Input: dimensioned drawing with shaded views. Units: mm. Origin: part minimum x, y, z. A direction names the side the tool comes from. Coordinates: 2 decimals unless noted, no trailing zeros. Order: outer loops, then holes, each group sorted by start corner. A loop starts at its lowest first (then second) coordinate and runs counter-clockwise, first axis right, second up.
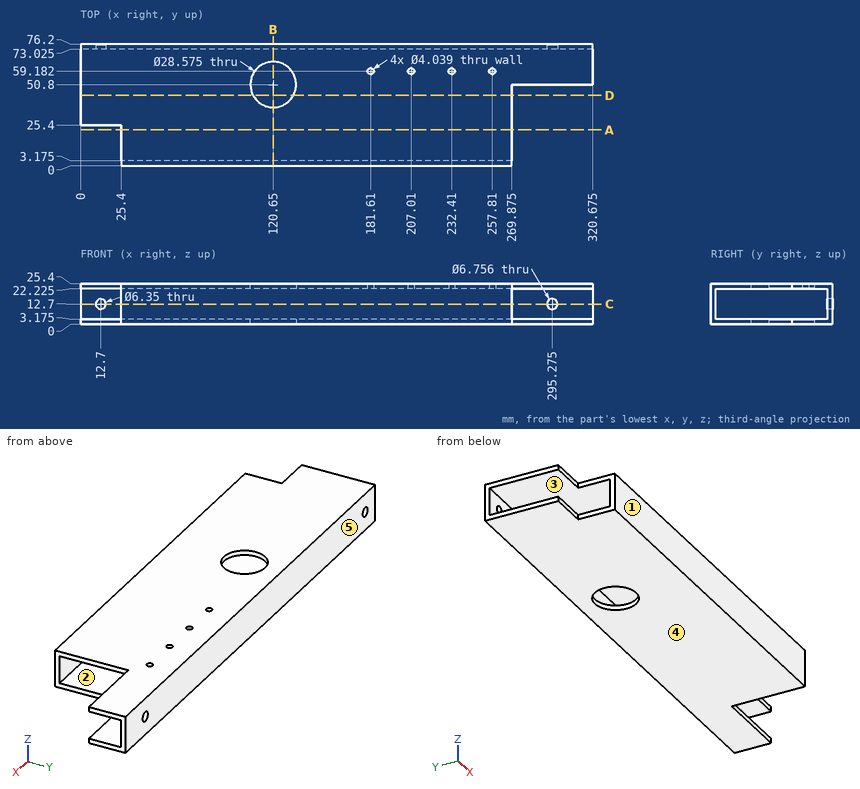
1. Section query B-B on x = 120.65. Return loops of the section in (y, z) (1 decimal).
Findings:
outline: (0, 0) - (36.5, 0) - (36.5, 3.2) - (3.2, 3.2) - (3.2, 22.2) - (36.5, 22.2) - (36.5, 25.4) - (0, 25.4) - close; (65.1, 0) - (76.2, 0) - (76.2, 25.4) - (65.1, 25.4) - (65.1, 22.2) - (73, 22.2) - (73, 3.2) - (65.1, 3.2) - close
2. Access query for the marked faces 1 and 2. Directions: +Z, -Z, +X, -X, +Y, -Y. A direction counts if a zero-diameter tool reaches every point of the face in a straight line with its end or side. Return the directions, or none.
Findings:
face 1: +Z, -Z, +X, -X, -Y
face 2: +X, -X
3. Pin query (flat end, axial travel): P1, Ø1.6, axis at x = 304.5, z = 23.5, coming from the -Y side; P2, Ø2.5, axis at x = 11.5, z = 24, coming from the -Y side; P3, Ø1, axis at y = 16.5, z = 22, coming from the +X side (3 decimals). Return the tip coordinate at first contact, or that it passes through.
Findings:
P1: stops at y = 50.8
P2: stops at y = 25.4
P3: stops at x = 269.875
4. Section query C-C on z = 12.7. Return loops of the section in (x, y) (1 decimal), plus the area to 3 significant figures.
Findings:
outline: (0, 73) - (9.5, 73) - (9.5, 76.2) - (0, 76.2) - close; (15.9, 73) - (291.9, 73) - (291.9, 76.2) - (15.9, 76.2) - close; (25.4, 0) - (269.9, 0) - (269.9, 3.2) - (25.4, 3.2) - close; (298.7, 73) - (320.7, 73) - (320.7, 76.2) - (298.7, 76.2) - close
area: 1,750 mm2
5. Section query A-A on y = 22.5. Return loops of the section in (x, z) (1 decimal).
Findings:
outline: (25.4, 0) - (269.9, 0) - (269.9, 3.2) - (25.4, 3.2) - close; (25.4, 22.2) - (269.9, 22.2) - (269.9, 25.4) - (25.4, 25.4) - close
6. Section query D-D on y = 44. Return loops of the section in (x, z) (1 decimal).
Findings:
outline: (0, 0) - (108.1, 0) - (108.1, 3.2) - (0, 3.2) - close; (0, 22.2) - (108.1, 22.2) - (108.1, 25.4) - (0, 25.4) - close; (133.2, 0) - (269.9, 0) - (269.9, 3.2) - (133.2, 3.2) - close; (133.2, 22.2) - (269.9, 22.2) - (269.9, 25.4) - (133.2, 25.4) - close
7. Ray query, line 1 (Y direction, x = 232.41, z = 24.1); line 2 (Y direction, x = 120.65, z = 24.15); line 3 (Z direction, x = 84.5, y = 51) (1 decimal). Return the intervals inside material, ascending.
Findings:
line 1: y = 0 to 57.16, 61.2 to 76.2
line 2: y = 0 to 36.51, 65.09 to 76.2
line 3: z = 0 to 3.2, 22.2 to 25.4
8. Draft query along Y for the marked faces 3, 4 and 5. Return one class per face: released by +Y, released by -Y, zero draft, split by the parting line, or undercut.
Findings:
face 3: undercut
face 4: zero draft
face 5: released by +Y
